Build history of the part. All positions in model axes, mm. A direction names the side the tool comes from. Coordinates: 2 decimals unless noted, no trailing zeros. Loops run counter-clockwise (first coordinate to the right, second up) from the corner with the lowest first, then second, coordinate; pieces in that order, holes last.
(1) Slice it at D-D (x = 458). Give the cut face in (y, z).
(2) Wall check: L1, parallel to X at y = 28.5, z = 69.5; L2, parallel to X at y = 68.5, z = 65; L3, parallel to X at y = 123.5, z = 40.5. Give the ranges that are in metal, low to high.
(3) Flat gauge pins, fed straight in: P1, Ø13.5, axis at y = 114, z = 25, coming from the +X side; P2, Ø2, axis at y = 20.5, z = 51, coming from the -X side. Where does each tip first touch, or does it go through?
(4) Tool access for faces 4 (the face through (869, 44.45, 45)), 5 (the face through (44, 95.25, 45)), 6 (the face through (387.35, 69, 66)), 7 (the face through (825.5, 117, 45)): list every direction of +Z, -Z, +X, -X, +Y, -Y with a clear straight run to the whole face (end or side of a thin tool).
(5) Slice it at A-A (z = 58.5). Give the cut face in (x, y), and give its area (3 significant figures).
(6) Slice it at C-C (y = 11.5). Give the cut face in (x, z).
(7) Slice it at B-B (y = 77). Give the cut face in (x, z).
(8) Two-plate mould, pull along X, no slides. Class faces 1 (the face through (825.5, 22, 45)), 2 (the face through (234, 71, 88.9)), 3 (the face through (527.05, 69, 66)): pulls with the +X half, pulls with the -X half, needs draft (parallel to the pull), parting line crosses it, or undercut.
from build123d import *

# Parameters (mm, degrees)
F0_W     = 914.4
F0_H     = 139.7
F1_DEPTH = 88.9
F2_W     = 88.9
F2_H     = 44.45
F3_DEPTH = 88.9
F4_W     = 139.7
F4_H     = 44.45
F5_DEPTH = 139.7


with BuildPart() as f1:
    # F0 (on Top) → F1 (new body)
    with BuildSketch(Plane.XY):
        with Locations((457.2, 69.85)):
            Rectangle(F0_W, F0_H)
    extrude(amount=F1_DEPTH)

    # F2 (on face) → F3 (cut, through all)
    with BuildSketch(Plane.XY.offset(88.9)):
        with Locations((44.45, 117.475)):
            Rectangle(F2_W, F2_H)
        with Locations((44.45, 22.225)):
            Rectangle(F2_W, F2_H)
        with Locations((869.95, 117.475)):
            Rectangle(F2_W, F2_H)
        with Locations((869.95, 22.225)):
            Rectangle(F2_W, F2_H)
    extrude(amount=-F3_DEPTH, mode=Mode.SUBTRACT)

    # F4 (on face) → F5 (cut, through all)
    with BuildSketch(Plane.XZ):
        with Locations((457.2, 66.675)):
            Rectangle(F4_W, F4_H)
    extrude(amount=-F5_DEPTH, mode=Mode.SUBTRACT)


solid = f1.part
Response values:
1. outline: (0, 0) - (139.7, 0) - (139.7, 44.45) - (0, 44.45) - close
2. L1: x = 88.9 to 387.35, 527.05 to 825.5
2. L2: x = 0 to 387.35, 527.05 to 914.4
2. L3: x = 88.9 to 825.5
3. P1: stops at x = 825.5
3. P2: stops at x = 88.9
4. face 4: +Z, -Z, +X, -Y
4. face 5: +Z, -Z, -X, +Y
4. face 6: +Z, +Y, -Y
4. face 7: +Z, -Z, +X, +Y
5. outline: (0, 44.45) - (88.9, 44.45) - (88.9, 0) - (387.35, 0) - (387.35, 139.7) - (88.9, 139.7) - (88.9, 95.25) - (0, 95.25) - close; (527.05, 0) - (825.5, 0) - (825.5, 44.45) - (914.4, 44.45) - (914.4, 95.25) - (825.5, 95.25) - (825.5, 139.7) - (527.05, 139.7) - close
5. area: 92,400 mm2
6. outline: (88.9, 0) - (825.5, 0) - (825.5, 88.9) - (527.05, 88.9) - (527.05, 44.45) - (387.35, 44.45) - (387.35, 88.9) - (88.9, 88.9) - close
7. outline: (0, 0) - (914.4, 0) - (914.4, 88.9) - (527.05, 88.9) - (527.05, 44.45) - (387.35, 44.45) - (387.35, 88.9) - (0, 88.9) - close
8. face 1: pulls with the +X half
8. face 2: needs draft
8. face 3: undercut
